Geometry: see drawing. Coordinates: mm, zero at the bounding-box minimum. A direction names the side the tool comes from. Give positions to 0.01 mm unless a question says otherwise; leave off trailing zeros. Write each loop counter-clockwise with the first axis right and the second up, starting at its lowest first coordinate (ties: lowest second). Pieces come first, ordered by that corner, then holes. Notation, with made-up numbers: (-38, 17) -> (-2, 17) arc R13 ccw to (-2, 42) -> close; hole circle Ø5 at (-24.5, 28.25). An arc over 180 degrees is marked (long way). Write item = value, one per line.
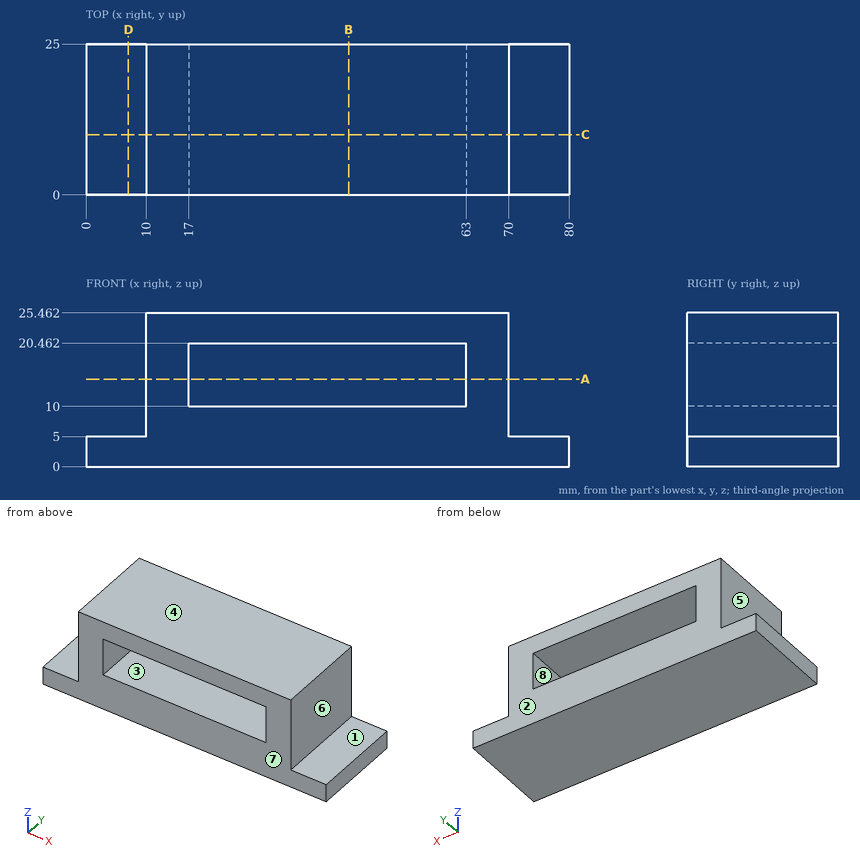
(1) Material intervals for line 1 (X direction, y = 22.25, z = 15.25); line 2 (Z direction, x = 46, y = 22.25); line 3 (X direction, y = 23.25, z = 21), sorted ascending.
Values follow:
line_1 = 10 to 17, 63 to 70
line_2 = 0 to 10, 20.46 to 25.46
line_3 = 10 to 70
(2) Section query B-B (x = 43.5). Return loops of the section in (y, z).
Values follow:
outline = (0, 0) -> (25, 0) -> (25, 10) -> (0, 10) -> close; (0, 20.46) -> (25, 20.46) -> (25, 25.46) -> (0, 25.46) -> close
(3) Section query C-C (y = 10). Return loops of the section in (x, z), plus the area to 3 significant figures.
Values follow:
outline = (0, 0) -> (80, 0) -> (80, 5) -> (70, 5) -> (70, 25.46) -> (10, 25.46) -> (10, 5) -> (0, 5) -> close; hole (17, 10) -> (63, 10) -> (63, 20.46) -> (17, 20.46) -> close
area = 1,150 mm2
(4) Access query for the marked faces 1, 2, 3, 4 and 5. Directions: +Z, -Z, +X, -X, +Y, -Y. A direction counts if a zero-diameter tool reaches every point of the face in a straight line with its end or side. Return the directions, or none.
Values follow:
face_1 = +Z, +X, +Y, -Y
face_2 = +Z, -Z, +X, -X, +Y
face_3 = +Y, -Y
face_4 = +Z, +X, -X, +Y, -Y
face_5 = +Z, -X, +Y, -Y
(5) Pull-direction query (X, two-part tool) for the marked faces 6, 7 and 8; classes: pulls with the +X half, pulls with the -X half, needs draft (parallel to the pull), parting line crosses it, or undercut.
Values follow:
face_6 = pulls with the +X half
face_7 = needs draft
face_8 = undercut
(6) First-contact query: pin 1 (5 mm diameter, centred on y = 13, z = 13, fed in from +X); pin 2 (6 mm diameter, centred on x = 42, y = 12, fed in from -Z); pin 3 (5 mm diameter, centred on x = 7, y = 10, fed in from +Z); pin 4 (2 mm diameter, centred on y = 13, z = 21, fed in from -X). Flat tips, straight axial feed; report the tip coordinate or a pass-through.
Values follow:
pin_1 = 70
pin_2 = 0
pin_3 = 5
pin_4 = 10
(7) Section query D-D (x = 7). Return loops of the section in (y, z), plus the area to 3 significant figures.
Values follow:
outline = (0, 0) -> (25, 0) -> (25, 5) -> (0, 5) -> close
area = 125 mm2
(8) Section query A-A (z = 14.5). Return loops of the section in (x, y).
Values follow:
outline = (10, 0) -> (17, 0) -> (17, 25) -> (10, 25) -> close; (63, 0) -> (70, 0) -> (70, 25) -> (63, 25) -> close
